Input: part model. Units: mm. Frame: model coordinates. A direction names the side the tool comes from. Coordinates: 2 decimals unless noted, no trailing zeros. Loops run counter-clockwise (first coordinate to the right, second up) from the corner with the lowest first, then second, coordinate; pieces in that order, holes last.
Item 1: Section A-A on y = 1. Return loops of the section in (x, z) (1 decimal).
Item 2: Contact query for flat-ended pins moving along their axis: P1, Ø2, axis at x = 1.5, z = 1.5, coming from the -Y side; P2, Ø0.7, axis at x = -0.5, z = -0.5, coming from the -Y side. Output: stop coordinate, or through.
Item 3: Ray query, line 1 along Y through (x, z) = (-0.7, -1.6); line 2 along Y through (x, z) = (-0.3, -0.85); line 3 along Z through (x, y) = (0.1, 4.5). Return the intervals inside material, ascending.
Item 4: Section C-C on z = 0.2. Return loops of the section in (x, y).
Item 5: Reachability of faces 1 (the flat face through (1.06, 0.81, -0.63)), 2 (the cylindrical face through (-1.5, 10.89, -0.07)), 3 (the flat face through (1.1, 0, 1.1)) from +Z, -Z, +X, -X, +Y, -Y: full face, straight path, thin tool, end or side. Return the list, or none.
Item 6: Pull-direction query (X, two-part tool) for faces 4 (the flat face through (1.074, 0.813, 0.608)), 5 (the flat face through (-1.074, 0.813, -0.608)), 6 (the flat face through (0, 3, 2)), 7 (the cylindrical face through (-0.54, 1.48, 2.44)); classes: released by +X, released by -X, zero draft, split by the parting line, or undercut.
Item 7: Section B-B on x = 0. Return loops of the section in (y, z), and give its area (3 significant figures).
Item 8: Section D-D on y = 16.25. Return loops of the section in (x, z).
```python
from build123d import *

# Parameters (mm, degrees)
SKETCH_1_R          = 2.5
EXTRUDE_1_DEPTH     = 3
SKETCH_2_R          = 1.5
EXTRUDE_2_DEPTH     = 16
CUT_EXTRUDE_1_DEPTH = 1.65


with BuildPart() as part:
    # 草图1 → 凸台-拉伸1 (new body)
    with BuildSketch(Plane(origin=(0, 0, 0), x_dir=(1, 0, 0), z_dir=(0, 1, 0))):
        Circle(SKETCH_1_R)
    extrude(amount=EXTRUDE_1_DEPTH)

    # 草图2 → 凸台-拉伸2 (add)
    with BuildSketch(Plane(origin=(0, 3, 0), x_dir=(1, 0, 0), z_dir=(0, 1, 0))):
        Circle(SKETCH_2_R)
    extrude(amount=EXTRUDE_2_DEPTH)

    # 草图3 → 切除-拉伸1 (cut)
    with BuildSketch(Plane.XZ):
        Polygon((1.425, 0), (0.7125, 1.2340862), (-0.7125, 1.2340862), (-1.425, 0), (-0.7125, -1.2340862), (0.7125, -1.2340862), align=None)
    extrude(amount=-CUT_EXTRUDE_1_DEPTH, mode=Mode.SUBTRACT)


solid = part.part
```
Results found:
1. outline: circle Ø5 at (0, 0); hole (-1.4, 0) - (-0.7, -1.2) - (0.7, -1.2) - (1.4, 0) - (0.7, 1.2) - (-0.7, 1.2) - close
2. P1: stops at y = 0
2. P2: stops at y = 1.65
3. line 1: y = 0 to 3
3. line 2: y = 1.65 to 19
3. line 3: z = -1.5 to 1.5
4. outline: (-2.49, 0) - (-1.31, 0) - (-1.31, 1.65) - (1.31, 1.65) - (1.31, 0) - (2.49, 0) - (2.49, 3) - (1.49, 3) - (1.49, 19) - (-1.49, 19) - (-1.49, 3) - (-2.49, 3) - close
5. face 1: -Y
5. face 2: +Y
5. face 3: +Z, -Z, +X, -X, -Y
6. face 4: undercut
6. face 5: undercut
6. face 6: zero draft
6. face 7: split by the parting line
7. outline: (0, -2.5) - (3, -2.5) - (3, -1.5) - (19, -1.5) - (19, 1.5) - (3, 1.5) - (3, 2.5) - (0, 2.5) - (0, 1.23) - (1.65, 1.23) - (1.65, -1.23) - (0, -1.23) - close
7. area: 58.9 mm2
8. outline: circle Ø3 at (0, 0)
